Input: part model. Units: mm. Frame: model coordinates. Face numbers are marked on the shaded views. A direction names the side the tool comes from. Coordinates: 2 decimals unless noted, no trailing zeros. Order: outer loops, then holes, each group sorted by start corner. A loop starts at its lowest first (then second) coordinate and runs counter-clockwise, first axis right, second up. Notation, with made-up numbers: M 50,27.25 L 57,27.25 A34 ccw 57,66.25 Z; hole C 4,86 d1. An arc over 180 degrees is marked long. One line per item, written item: value.
```python
from build123d import *

# Parameters (mm, degrees)
F0_R     = 45
F0_R_2   = 25
F1_DEPTH = 34
F2_SIZE  = 2
F3_SIZE  = 2
F4_SIZE  = 2
F5_R     = 37.775597
F5_R_2   = 31.34905
F6_DEPTH = 1
F7_R     = 37.775597
F7_R_2   = 31.34905
F8_DEPTH = 1


with BuildPart() as f1:
    # F0 (on Front) → F1 (new body)
    with BuildSketch(Plane.XZ):
        Circle(F0_R)
        Circle(F0_R_2, mode=Mode.SUBTRACT)
    extrude(amount=F1_DEPTH)

    # F2
    f2_edges = [f1.edges().sort_by_distance(p)[0] for p in [
        (-45, -34, 0),
        (-45, 0, 0),
    ]]
    chamfer(f2_edges, length=F2_SIZE)

    # F3
    f3_edges = [f1.edges().sort_by_distance(p)[0] for p in [
        (-25, -34, 0),
    ]]
    chamfer(f3_edges, length=F3_SIZE)

    # F4
    f4_edges = [f1.edges().sort_by_distance(p)[0] for p in [
        (-25, 0, 0),
    ]]
    chamfer(f4_edges, length=F4_SIZE)

    # F5 (on face) → F6 (cut)
    with BuildSketch(Plane(origin=(0, 0, 0), x_dir=(-1, 0, 0), z_dir=(0, 1, 0))):
        Circle(F5_R)
        Circle(F5_R_2, mode=Mode.SUBTRACT)
    extrude(amount=-F6_DEPTH, mode=Mode.SUBTRACT)

    # F7 (on face) → F8 (cut)
    with BuildSketch(Plane.XZ.offset(34)):
        Circle(F7_R)
        Circle(F7_R_2, mode=Mode.SUBTRACT)
    extrude(amount=-F8_DEPTH, mode=Mode.SUBTRACT)


solid = f1.part
```
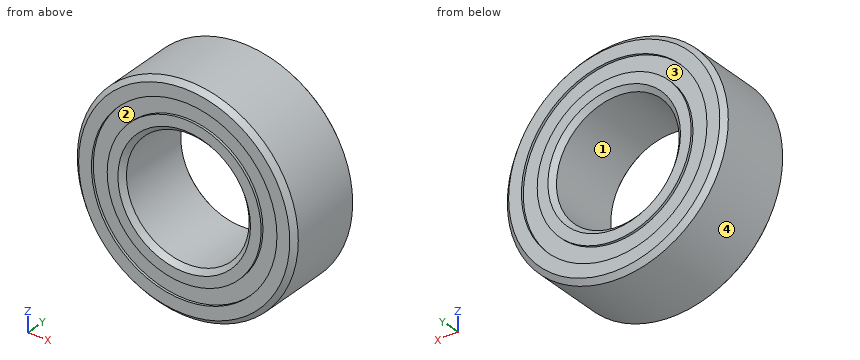
(1) First-contact query: pin 1 (5 mm diameter, centred on x = 31.5, y = -9.5, fed in from +Z); pin 2 (1.5 mm diameter, centred on x = -9, z = -34.5, fed in from +Y); pin 3 (10 mm diameter, centred on y = -17, z = -22, fed in from -X); pin 4 (4 mm diameter, centred on x = -17.5, z = 12, fed in from +Y). Flat tips, straight axial feed; report the tip coordinate or a pass-through.
Data:
pin 1: stops at z = 34.41
pin 2: stops at y = -1
pin 3: stops at x = -41.67
pin 4: passes through
(2) Access query for the marked faces 1 and 2. Directions: +Z, -Z, +X, -X, +Y, -Y. A direction counts if a zero-diameter tool reaches every point of the face in a straight line with its end or side. Return the directions, or none.
Data:
face 1: +Y, -Y
face 2: -Y
(3) Cut plane C-C on y = -15.5. Output: boundary loops of the cut face in (x, z), plus the area to 3 significant figures.
Data:
outline: C 0,0 d90; hole C 0,0 d50
area: 4,400 mm2
(4) Draft query along Z for the marked faces 3 and 4. Return one class per face: released by +Z, released by -Z, zero draft, split by the parting line, or undercut.
Data:
face 3: undercut
face 4: split by the parting line
(5) Ray query, line 1 (X direction, y = -20, z = -36); line 2 (Z direction, x = -20, y = -15); line 3 (Z direction, x = 0, y = -33.4). Return the intervals inside material, ascending. Write a range as from..to.
Data:
line 1: x = -27..27
line 2: z = -40.31..-15, 15..40.31
line 3: z = -43.6..-37.78, -31.35..-26.4, 26.4..31.35, 37.78..43.6
